Work out the finished part from the listing and answer in its coordinate system (mm). A direction names the side the tool comes from. Coordinates: 2 decimals unless noted, no trailing zeros. Loops run counter-clockwise (first coordinate to the right, second up) from the corner with the lowest first, then second, coordinate; pieces in that order, holes last. Notation, with made-up numbers: (74.5, 10.5) -> (117.5, 10.5) arc R29 ccw to (117.5, 33.5) -> close; hole circle Ø6 at (8, 61.25). An arc over 180 degrees is marked (long way). Answer as CSV lines item,"result".
Autodesk Inventor part; units mm, degrees
ref_plane "YZ Plane" through (0, 0, 0) normal (1, 0, 0) x (0, 1, 0)
ref_plane "XZ Plane" through (0, 0, 0) normal (0, 1, 0) x (-1, 0, 0)
ref_plane "XY Plane" through (0, 0, 0) normal (0, 0, 1) x (1, 0, 0)
sketch "Esquisse3" plane through (0, 0, 0) normal (0, 0, 1) x (1, 0, 0)
  line L0 (41.5, -212.5) -> (-41.5, -212.5)
  line L1 (-41.5, -212.5) -> (-41.5, 212.5)
  line L2 (-41.5, 212.5) -> (41.5, 212.5)
  line L3 (41.5, 212.5) -> (41.5, -212.5)
  line L4 (41.5, -212.5) -> (-41.5, 212.5) construction
  line L5 (-41.5, -212.5) -> (41.5, 212.5) construction
  point P0 (0, 0)
  dimension "d20" = 83
  dimension "d21" = 425
extrude "Extrusion3" add sketch "Esquisse3" along normal blind 18.55
sketch "Esquisse4" plane through (0, 0, 18.55) normal (0, 0, 1) x (1, 0, 0)
  line L0 (41.5, 212.5) -> (22.9, 212.5)
  line L1 (22.9, 212.5) -> (22.9, 162.5)
  line L2 (22.9, 162.5) -> (41.5, 162.5)
  line L3 (41.5, 162.5) -> (41.5, 212.5)
  line L4 (-41.5, -212.5) -> (41.5, -212.5)
  line L5 (41.5, -212.5) -> (22.9, -212.5)
  line L6 (22.9, -212.5) -> (22.9, -137.5)
  line L7 (22.9, -137.5) -> (41.5, -137.5)
  line L8 (41.5, -137.5) -> (41.5, -212.5)
  line L9 (41.5, -37.5) -> (22.9, -37.5)
  line L10 (22.9, -37.5) -> (22.9, 62.5)
  line L11 (22.9, 62.5) -> (41.5, 62.5)
  line L12 (41.5, 62.5) -> (41.5, -37.5)
  point P0 (0, 0)
  dimension "d24" = 75
  dimension "d25" = 50
  dimension "d27" = 100
  dimension "d29" = 100
  dimension "d30" = 100
  dimension "d31" = 18.6
extrude "Extrusion4" cut sketch "Esquisse4" against normal blind 18.55
sketch "Esquisse5" plane through (0, 0, 18.55) normal (0, 0, 1) x (1, 0, 0)
  line L0 (22.9, 212.5) -> (-41.5, 212.5)
  line L1 (-41.5, 212.5) -> (-22.95, 212.5)
  line L2 (-22.95, 212.5) -> (-22.95, 192.5)
  line L3 (-22.95, 192.5) -> (-41.5, 192.5)
  line L4 (-41.5, 192.5) -> (-41.5, 212.5)
  line L5 (-41.5, 212.5) -> (-41.5, -212.5)
  line L6 (-41.5, 122.5) -> (-22.95, 122.5)
  line L7 (-22.95, 122.5) -> (-22.95, 41.5)
  line L8 (-22.95, 41.5) -> (-41.5, 41.5)
  line L9 (-41.5, 41.5) -> (-41.5, 122.5)
  line L10 (-41.5, -28.5) -> (-22.95, -28.5)
  line L11 (-22.95, -28.5) -> (-22.95, -212.5)
  line L12 (-22.95, -212.5) -> (-41.5, -212.5)
  line L13 (-41.5, -212.5) -> (-41.5, -28.5)
  line L14 (-41.5, -212.5) -> (22.9, -212.5)
  point P0 (0, 0)
  point P1 (-41.5, 41.5)
  dimension "d34" = 20
  dimension "d35" = 18.55
  dimension "d37" = 70
  dimension "d38" = 81
  dimension "d39" = 70
extrude "Extrusion5" cut sketch "Esquisse5" against normal blind 18.55
sketch "Esquisse6" plane through (0, 0, 18.55) normal (0, 0, 1) x (1, 0, 0)
  circle A0 centre (-24.0708, 193.6208) radius 1.585
  circle A1 centre (24.0208, 163.6208) radius 1.585
  circle A2 centre (-24.0708, 121.3792) radius 1.585
  circle A3 centre (24.0208, 61.3792) radius 1.585
  circle A4 centre (-24.0708, 42.6208) radius 1.585
  circle A5 centre (24.0208, -36.3792) radius 1.585
  circle A6 centre (-24.0708, -29.6208) radius 1.585
  circle A7 centre (24.0208, -138.6208) radius 1.585
  line L0 (-41.5, 192.5) -> (-22.95, 192.5)
  line L1 (-24.0708, 193.6208) -> (-22.95, 192.5) construction
  line L2 (41.5, 162.5) -> (22.9, 162.5)
  line L3 (22.9, 162.5) -> (24.0208, 163.6208) construction
  line L4 (-22.95, 122.5) -> (-41.5, 122.5)
  line L5 (-22.95, 122.5) -> (-24.0708, 121.3792) construction
  line L6 (-24.0708, 42.6208) -> (-22.95, 41.5) construction
  line L7 (-41.5, 41.5) -> (-22.95, 41.5)
  line L8 (22.9, 62.5) -> (24.0208, 61.3792) construction
  line L9 (-22.95, -28.5) -> (-41.5, -28.5)
  line L10 (-22.95, -28.5) -> (-24.0708, -29.6208) construction
  line L11 (-22.95, -28.5) -> (-22.95, -212.5)
  line L12 (41.5, -37.5) -> (22.9, -37.5)
  line L13 (22.9, -37.5) -> (24.0208, -36.3792) construction
  line L14 (22.9, -37.5) -> (22.9, 62.5)
  line L15 (22.9, -137.5) -> (41.5, -137.5)
  line L16 (22.9, -137.5) -> (24.0208, -138.6208) construction
  point P0 (0, 0)
  dimension "d43" = 3.17
  dimension "d46" = 45
  dimension "d47" = 45
  dimension "d49" = 45
  dimension "d51" = 45
  dimension "d52" = 45
  dimension "d53" = 45
  dimension "d54" = 45
extrude "Extrusion6" cut sketch "Esquisse6" against normal blind 18.55
properties part number "cover"
(1) A cutting plane is placed at D-D, the plane y = -24. Write down the section's boundary in (x, z), and give its area (3 significant figures).
Computed values:
outline,"(-41.5, 0) -> (22.9, 0) -> (22.9, 18.55) -> (-41.5, 18.55) -> close"
area,"1,190 mm2"
(2) Which of the six approach directions +Z, -Z, +X, -X, +Y, -Y give full straight-line access (tool end or side, diameter ignored) to faces 5 (the face through (-22.95, -120, 9)), 6 (the face through (33, 62.5, 9)), 7 (the face through (-33, 122.5, 9)), 8 (the face through (22.9, 189, 9)), 9 (the face through (-33, 192.5, 9))?
Computed values:
face 5,"+Z, -Z, -X, -Y"
face 6,"+Z, -Z, +X"
face 7,"+Z, -Z, -X"
face 8,"+Z, -Z, +X, +Y"
face 9,"+Z, -Z, -X, +Y"
(3) A cutting plane is placed at A-A, the plane x = -36. Write down the section's boundary in (y, z).
Computed values:
outline,"(-28.5, 0) -> (41.5, 0) -> (41.5, 18.55) -> (-28.5, 18.55) -> close; (122.5, 0) -> (192.5, 0) -> (192.5, 18.55) -> (122.5, 18.55) -> close"
(4) For a pull along Y with two mould halves and no side action, classify faces 1 (the face through (33, -137.5, 9)), 2 (the face through (33, 162.5, 9)), 3 (the face through (-41.5, 6, 9)), 4 (the face through (-22.95, 83, 9)) as pulls with the +Y half, pulls with the -Y half, needs draft (parallel to the pull), parting line crosses it, or undercut.
Computed values:
face 1,"pulls with the -Y half"
face 2,"pulls with the +Y half"
face 3,"needs draft"
face 4,"undercut"
(5) A cutting plane is placed at C-C, the plane x = 33.5. Write down the section's boundary in (y, z), and give its area (3 significant figures).
Computed values:
outline,"(-137.5, 0) -> (-37.5, 0) -> (-37.5, 18.55) -> (-137.5, 18.55) -> close; (62.5, 0) -> (162.5, 0) -> (162.5, 18.55) -> (62.5, 18.55) -> close"
area,"3,710 mm2"
(6) A cutting plane is placed at B-B, the plane z = 4. Write down the section's boundary in (x, y) (3 decimals), and give its area (3 significant figures).
Computed values:
outline,"(-41.5, -28.5) -> (-25.192, -28.5) arc R1.585 cw to (-22.95, -30.742) -> (-22.95, -212.5) -> (22.9, -212.5) -> (22.9, -139.742) arc R1.585 cw to (25.142, -137.5) -> (41.5, -137.5) -> (41.5, -37.5) -> (25.142, -37.5) arc R1.585 cw to (22.9, -35.258) -> (22.9, 60.258) arc R1.585 cw to (25.142, 62.5) -> (41.5, 62.5) -> (41.5, 162.5) -> (25.142, 162.5) arc R1.585 cw to (22.9, 164.742) -> (22.9, 212.5) -> (-22.95, 212.5) -> (-22.95, 194.742) arc R1.585 cw to (-25.192, 192.5) -> (-41.5, 192.5) -> (-41.5, 122.5) -> (-25.192, 122.5) arc R1.585 cw to (-22.95, 120.258) -> (-22.95, 43.742) arc R1.585 cw to (-25.192, 41.5) -> (-41.5, 41.5) -> close"
area,"25,800 mm2"
(7) Consider line 1 along Y through (x, z) = (-34.5, 14); line 2 along Y through (x, z) = (-24, 2.75); line 3 along X through (y, z) = (-43, 17.75). Determine where each line is inside the solid, lowest interval first.
Computed values:
line 1,"-28.5 to 41.5, 122.5 to 192.5"
line 2,"-28.04 to 41.04, 122.96 to 192.04"
line 3,"-22.95 to 41.5"
(8) Flat-ended cylindrical pins translate along their axes: pin 1 Ø3 at (x, z) = (-28.5, 4.5) entering from -Y; pin 2 Ø8 at (x, z) = (31.5, 13.5) entering from +Y; pin 3 Ø4 at (y, z) = (-142.5, 16.5) entering from +X. Find the tip coordinate at first contact, or state that the pin passes through.
Computed values:
pin 1,"y = -28.5"
pin 2,"y = 162.5"
pin 3,"x = 22.9"
